Read the model definition and answer for the solid it produces. Units are mm, in the model's axes. A direction names the side the tool comes from. Give positions to 0.01 mm unless a question says otherwise; leave off trailing zeros. Order: outer loops, then holes, each group sorted by start corner. A loop starts at its lowest first (then second) coordinate and runs counter-clockwise, first axis right, second up. Notation, with made-up numbers: M 59,-1.5 L 70,-1.5 A17 ccw 70,17.5 Z; hole C 69.5,-12.75 d5. An arc over 180 degrees is marked long. One line per item, written item: value.
from build123d import *

# Parameters (mm, degrees)
F2_R     = 7.31
F3_DEPTH = 1.8
F4_R     = 5


with BuildPart() as f1:
    # F0 (on Top) → F1 (revolve)
    with BuildSketch(Plane.XY):
        Polygon((91.7, 8.25), (9.2, 8.25), (6.95, 2.4), (0, 2), (0, 1.300344), (7.704519, 1.74377), (9.845377, 7.31), (91.7, 7.31), align=None)
    revolve(axis=Axis((40.51489, 0, 0), (1, 0, 0)))

    # F2 (on face) → F3 (join)
    with BuildSketch(Plane.YZ.offset(91.7)):
        Polygon((-14.5, 6), (-14.5, 0), (-14.5, -6), (0, -10), (14.5, -6), (14.5, 0), (14.5, 6), (0, 10), align=None)
        Circle(F2_R, mode=Mode.SUBTRACT)
    extrude(amount=F3_DEPTH)

    # F4
    f4_edges = [f1.edges().sort_by_distance(p)[0] for p in [
        (92.6, -14.5, 6),
        (92.6, -14.5, -6),
        (92.6, 0, -10),
        (92.6, 14.5, -6),
        (92.6, 14.5, 6),
        (92.6, 0, 10),
    ]]
    fillet(f4_edges, radius=F4_R)


solid = f1.part
1) Determine the mould class of faces 3 (the face through (92.613, -13.505, -5.185)), 4 (the face through (51.09, -0.95, 7.25)), 5 (the face through (92.613, 13.505, 5.185)) for opening direction Y: +Y half, -Y half, draft (parallel to the pull), parting line (faces both ways), or undercut.
Reported:
face 3: -Y half
face 4: undercut
face 5: +Y half
2) Find section B-B, the plane z = 0. Write down the section's boundary in (x, y), plus the area to 3 significant figures.
Reported:
outline: M 0,-2 L 6.95,-2.4 L 9.2,-8.25 L 91.7,-8.25 L 91.7,-14.5 L 93.5,-14.5 L 93.5,-7.31 L 9.85,-7.31 L 7.7,-1.74 L 0,-1.3 Z; M 0,1.3 L 7.7,1.74 L 9.85,7.31 L 93.5,7.31 L 93.5,14.5 L 91.7,14.5 L 91.7,8.25 L 9.2,8.25 L 6.95,2.4 L 0,2 Z
area: 202 mm^2
3) Which of the six approach directions +Z, -Z, +X, -X, +Y, -Y give full straight-line access (tool end or side, diameter ignored) to faces 1 (the face through (91.7, 0, -9)), 2 (the face through (3.91, -1.21, -0.93))?
Reported:
face 1: -X
face 2: +X
4) Each of these flat-tipped pins is pushed along its axis until it touches: pin 1 Ø10 at (x, z) = (10.5, -0.5) entering from -Y; pin 2 Ø2 at (x, z) = (61, -0.5) entering from +Y; pin 3 Ø6 at (x, y) = (67.5, 3) entering from -Z. Where does it stop, or does it pass through?
Reported:
pin 1: stops at y = -8.25
pin 2: stops at y = 8.25
pin 3: stops at z = -8.25
5) Find section C-C, the plane x = 60. Write down the section's boundary in (y, z), plus the area to 3 significant figures.
Reported:
outline: C 0,0 d16.5; hole C 0,0 d14.62
area: 46.0 mm^2
6) Consider probe 1 along Z at (x, y) = (73, 0); probe 2 along Y at (x, z) = (42, 3.75); probe 3 along Y at (x, z) = (71.5, 4.5). Determine where each line is inside the solid, lowest interval first.
Reported:
probe 1: z = -8.25 to -7.31, 7.31 to 8.25
probe 2: y = -7.35 to -6.27, 6.27 to 7.35
probe 3: y = -6.91 to -5.76, 5.76 to 6.91
7) Find section A-A, the plane y = 0. Write down the section's boundary in (x, z), plus the area to 3 significant figures.
Reported:
outline: M 0,-2 L 6.95,-2.4 L 9.2,-8.25 L 91.7,-8.25 L 91.7,-9.81 L 93.5,-9.81 L 93.5,-7.31 L 9.85,-7.31 L 7.7,-1.74 L 0,-1.3 Z; M 0,1.3 L 7.7,1.74 L 9.85,7.31 L 93.5,7.31 L 93.5,9.81 L 91.7,9.81 L 91.7,8.25 L 9.2,8.25 L 6.95,2.4 L 0,2 Z
area: 185 mm^2
